Geometry check sheet. Reference: the model listing, model coordinates, mm. Face numbers are marked on the shaded views. A direction names the side the tool comes from. Coordinates: 2 decimals unless noted, no trailing zeros. Loops run counter-clockwise (first coordinate to the right, second up) from the corner with the lowest first, then second, coordinate; pieces in that order, holes last. Notation, with made-up numbers: M -36,43.25 L -27,43.25 A22 ccw -27,78.25 Z; hole C 76,27 d4. An arc over 180 degrees is marked long. Use CSV: the item, a comma, the result in double quotes.
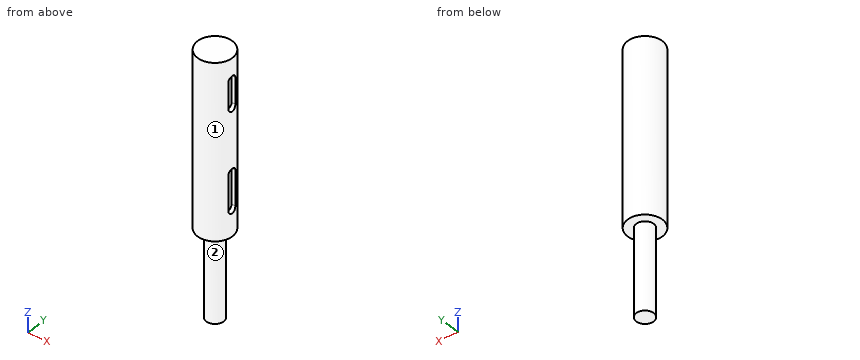
```python
from build123d import *

# Parameters (mm, degrees)
SKETCH_1_R          = 4
EXTRUDE_1_DEPTH     = 40
SKETCH_2_R          = 2
EXTRUDE_2_DEPTH     = 20
CUT_EXTRUDE_1_DEPTH = 2


with BuildPart() as part:
    # ｽｹｯﾁ1 → ﾎﾞｽ - 押し出し1 (new body)
    with BuildSketch(Plane.XY):
        Circle(SKETCH_1_R)
    extrude(amount=EXTRUDE_1_DEPTH)

    # ｽｹｯﾁ2 → ﾎﾞｽ - 押し出し2 (add)
    with BuildSketch(Plane(origin=(0, 0, 0), x_dir=(-1, 0, 0), z_dir=(0, 0, -1))):
        Circle(SKETCH_2_R)
    extrude(amount=EXTRUDE_2_DEPTH)

    # ｽｹｯﾁ3 → ｶｯﾄ - 押し出し1 (cut, through all)
    with BuildSketch(Plane(origin=(3, 0, 0), x_dir=(0, 0, -1), z_dir=(1, 0, 0))):
        with BuildLine():
            Line((-35, 1), (-29, 1))
            ThreePointArc((-29, 1), (-28, 0), (-29, -1))
            Line((-29, -1), (-35, -1))
            ThreePointArc((-35, -1), (-36, 0), (-35, 1))
        make_face()
        with BuildLine():
            Line((-14.2, 1), (-6.2, 1))
            ThreePointArc((-6.2, 1), (-5.2, 0), (-6.2, -1))
            Line((-6.2, -1), (-14.2, -1))
            ThreePointArc((-14.2, -1), (-15.2, 0), (-14.2, 1))
        make_face()
    extrude(amount=CUT_EXTRUDE_1_DEPTH, mode=Mode.SUBTRACT)


solid = part.part
```
1. Section check A-A, the plane x = 0. Record the cut outline in (y, z), plus the area to 3 significant figures.
The answers:
outline,"M -4,0 L -2,0 L -2,-20 L 2,-20 L 2,0 L 4,0 L 4,40 L -4,40 Z"
area,"400 mm^2"
2. Section check B-B, the plane y = 0.5. Record the cut outline in (x, z).
The answers:
outline,"M -3.97,0 L -1.94,0 L -1.94,-20 L 1.94,-20 L 1.94,0 L 3.97,0 L 3.97,5.33 L 3,5.33 L 3,15.07 L 3.97,15.07 L 3.97,28.13 L 3,28.13 L 3,35.87 L 3.97,35.87 L 3.97,40 L -3.97,40 Z"
3. Section check D-D, the plane z = 12. Record the cut outline in (x, y), plus the area to 3 significant figures.
The answers:
outline,"M 3,-1 L 3,1 L 3.87,1 A4 ccw long 3.87,-1 Z"
area,"48.3 mm^2"
4. Set-up check for the marked faces 1 and 2: record each of +Z, -Z, +X, -X, +Y, -Y from which the full face is reachable in a straight line by a thin tool's end or side.
The answers:
face 1,"+Z, -Z"
face 2,"-Z"
5. Thickness scan on line 1 (Z direction, x = -2.75, y = 2.5); line 2 (X direction, y = -0.25, z = 20); line 3 (Y direction, x = 3.5, z = 11). Record the ranges inside material, lowest first. Write a range as [from, to].
The answers:
line 1,"[0, 40]"
line 2,"[-3.99, 3.99]"
line 3,"[-1.94, -1], [1, 1.94]"
6. Gauge pin test, flat ends, axial feed: P1, Ø2, axis at y = -0.5, z = 12, coming from the +X side; P2, Ø0.7, axis at x = 3.5, z = 33, coming from the +Y side; P3, Ø1, axis at x = 3.5, z = 9.5, coming from the -Y side. Record the tip position at first contact, or that the pin passes through.
The answers:
P1,"x = 3.87"
P2,"y = 2.47"
P3,"y = -2.65"
7. Section check C-C, the plane z = 4.5. Record the cut outline in (x, y).
The answers:
outline,"C 0,0 d8"
